from build123d import *

# Parameters (mm, degrees)
P_IDAT_VYSUNUT_M1_DEPTH  = 2
SKICA2_R                 = 1.75
ODEBRAT_VYSUNUT_M1_DEPTH = 10
SKICA3_W                 = 63
SKICA3_H                 = 10
P_IDAT_VYSUNUT_M2_DEPTH  = 4
SKICA4_R                 = 2.5
ODEBRAT_VYSUNUT_M2_DEPTH = 24
ODEBRAT_VYSUNUT_M3_DEPTH = 10
P_IDAT_VYSUNUT_M3_DEPTH  = 2


with BuildPart() as part:
    # Skica1 → Přidat vysunutím1 (new body)
    with BuildSketch(Plane.XY):
        Polygon((-31.5, 0), (31.5, 0), (31.5, 28), (60.5, 28), (60.5, 59.5), (-60.5, 59.5), (-60.5, 28), (-31.5, 28), align=None)
    extrude(amount=P_IDAT_VYSUNUT_M1_DEPTH)

    # Skica2 → Odebrat vysunutím1 (cut)
    with BuildSketch(Plane(origin=(0, 0, 0), x_dir=(-1, 0, 0), z_dir=(0, 0, -1))):
        with Locations((-56, 56.5)):
            Circle(SKICA2_R)
        with Locations((-56, 32.5)):
            Circle(SKICA2_R)
        with Locations((-27, 4.5)):
            Circle(SKICA2_R)
        with Locations((27, 4.5)):
            Circle(SKICA2_R)
        with Locations((56, 32.5)):
            Circle(SKICA2_R)
        with Locations((56, 56.5)):
            Circle(SKICA2_R)
    extrude(amount=-ODEBRAT_VYSUNUT_M1_DEPTH, mode=Mode.SUBTRACT)

    # Skica3 → Přidat vysunutím2 (add)
    with BuildSketch(Plane.XY):
        with Locations((0, 15)):
            Rectangle(SKICA3_W, SKICA3_H)
    extrude(amount=-P_IDAT_VYSUNUT_M2_DEPTH)

    # Skica4 → Odebrat vysunutím2 (cut)
    with BuildSketch(Plane(origin=(0, 0, -4), x_dir=(-1, 0, 0), z_dir=(0, 0, -1))):
        with Locations((17.5, 15)):
            Circle(SKICA4_R)
        with Locations((25.5, 15)):
            Circle(SKICA4_R)
        with Locations((-25.5, 15)):
            Circle(SKICA4_R)
        with Locations((-17.5, 15)):
            Circle(SKICA4_R)
    extrude(amount=-ODEBRAT_VYSUNUT_M2_DEPTH, mode=Mode.SUBTRACT)

    # Skica5 → Odebrat vysunutím3 (cut)
    with BuildSketch(Plane.XY.offset(2)):
        Polygon((40, 59.5), (-40, 59.5), (-25, 29.5), (25, 29.5), align=None)
    extrude(amount=-ODEBRAT_VYSUNUT_M3_DEPTH, mode=Mode.SUBTRACT)

    # Skica6 → Přidat vysunutím3 (add)
    with BuildSketch(Plane(origin=(0, 0, 0), x_dir=(-1, 0, 0), z_dir=(0, 0, -1))):
        Polygon((-25, 29.5), (-26.341640786, 32.183281573), (-22, 29.5), align=None)
        Polygon((25, 29.5), (26.341640786, 32.183281573), (22, 29.5), align=None)
    extrude(amount=-P_IDAT_VYSUNUT_M3_DEPTH)


solid = part.part
CAD build for the part. Positions are in the model's coordinates, mm. A direction names the side the tool comes from. Coordinates: 2 decimals unless noted, no trailing zeros. Write each loop counter-clockwise with the first axis right and the second up, starting at its lowest first coordinate (ties: lowest second). Pieces come first, ordered by that corner, then holes. Notation, with made-up numbers: (-19.75, -39.5) - (7.25, -39.5) arc R24 cw to (7.25, -17.5) - close; hole circle Ø1 at (-2.75, 12). An arc over 180 degrees is marked (long way). Use a Markdown table: item, result. Add a question column.
Item 1: Flat gauge pins, fed straight in: pin 1 (4 mm diameter, centred on x = 56, y = 32.5, fed in from -Z); pin 2 (1.5 mm diameter, centred on x = 43, z = -2.5, fed in from -Y); pin 3 (2 mm diameter, centred on x = -39.5, z = 1.5, fed in from -Y); pin 4 (8 mm diameter, centred on x = 25.5, y = 15, fed in from +Z). Where does each tip first touch, or does it go through?
Item 2: Band-saw the part on B-B, the plane x = -17.5. Give the cut face in (y, z), and give its area (3 significant figures).
Item 3: Band-saw the part on C-C, the plane y = 15. Give the cut face in (x, z), and give its area (3 significant figures).
Item 4: 3-axis set-ups, long thin cutter, end or side, ignore diameter. For faces 5 (the face through (33.1, 45.7, 1)), 6 (the face through (-1, 27, 0)), 7 (the face through (-57.617, 55.83, 0.986)): which of +Z, -Z, +X, -X, +Y, -Y reach the whole face in a straight line?
Item 5: Drill centre lines: L1, parallel to Y at x = 56, z = 1.5; L2, parallel to Y at x = 17.5, z = 0.8; L3, parallel to Y at x = 49.5, z = 0.05. Where is each one in solid material? Low to high. Write a range as from..to.
Item 6: Band-saw the part on A-A, the plane y = 44.5. Give the cut face in (x, z).
Item 7: Band-saw the part on D-D, the plane z = -2.9. Give the cut face in (x, y), and give its area (3 significant figures).
Item 8: Mould opens along Y. For faces 1 (the face through (0, 10, -2)), 2 (the face through (-1, 24, 2)), 3 (the face through (20, 15, -1)), 4 (the face through (0, 20, -2)) say: pulls with the +Y half, pulls with the -Y half, needs draft (parallel to the pull), parting line crosses it, or undercut.
Numbers:
| question | item | result |
|---|---|---|
| 1 | pin 1 | z = 0 |
| 1 | pin 2 | through |
| 1 | pin 3 | y = 28 |
| 1 | pin 4 | z = 2 |
| 2 | outline | (0, 0) - (10, 0) - (10, -4) - (12.5, -4) - (12.5, 2) - (0, 2) - close; (17.5, -4) - (20, -4) - (20, 0) - (29.5, 0) - (29.5, 2) - (17.5, 2) - close |
| 2 | area | 69.0 mm2 |
| 3 | outline | (-31.5, -4) - (-28, -4) - (-28, 2) - (-31.5, 2) - close; (-23, -4) - (-20, -4) - (-20, 2) - (-23, 2) - close; (-15, -4) - (15, -4) - (15, 2) - (-15, 2) - close; (20, -4) - (23, -4) - (23, 2) - (20, 2) - close; (28, -4) - (31.5, -4) - (31.5, 2) - (28, 2) - close |
| 3 | area | 258 mm2 |
| 4 | face 5 | +Z, -Z, +Y |
| 4 | face 6 | -Z, +X, -X, +Y |
| 4 | face 7 | +Z, -Z |
| 5 | L1 | 28..30.75, 34.25..54.75, 58.25..59.5 |
| 5 | L2 | 0..12.5, 17.5..29.5 |
| 5 | L3 | 28..59.5 |
| 6 | outline | (-60.5, 0) - (-32.5, 0) - (-32.5, 2) - (-60.5, 2) - close; (32.5, 0) - (60.5, 0) - (60.5, 2) - (32.5, 2) - close |
| 7 | outline | (-31.5, 10) - (31.5, 10) - (31.5, 20) - (-31.5, 20) - close; hole circle Ø5 at (-25.5, 15); hole circle Ø5 at (-17.5, 15); hole circle Ø5 at (17.5, 15); hole circle Ø5 at (25.5, 15) |
| 7 | area | 551 mm2 |
| 8 | face 1 | pulls with the -Y half |
| 8 | face 2 | needs draft |
| 8 | face 3 | undercut |
| 8 | face 4 | pulls with the +Y half |
